Could you check a few things on this model? Use its own coordinates, in mm. Give positions to 0.01 mm unless a question says otherwise; leave off trailing zeros. Loops run counter-clockwise (first coordinate to the right, second up) from the corner with the lowest first, then second, coordinate; pieces in that order, holes last. Notation, with made-up numbers: M 69,13.25 L 96,13.25 A25 ccw 96,50.25 Z; hole C 0.25,43.5 d4. An arc over 180 degrees is marked long. Return JSON: item names as keys, results as strings. Group by question number.
1. If we section it at C-C (z = 2.5): Write out the boundary of the cut face in (x, y).
2. Please list where these lines run through material, in increasing order: line 1 (Y direction, x = 0, z = 1.2); line 2 (Z direction, x = 2.75, y = -1.75); line 3 (Y direction, x = -1.25, z = 0.75).
3. If we section it at D-D (z = 4.5): Write out the boundary of the cut face in (x, y).
4. For pin 1 (1.5 mm diameter, centred on y = -4, z = 2, fed in from -X); pin 2 (2.5 mm diameter, centred on x = -2, y = -1.5, fed in from +Z); pin 3 (1 mm diameter, centred on x = -3, z = 6.5, fed in from -Y), each with a flat end and sliding along its axis, tell me the tip position at first contact or that it passes through.
5. If we section it at A-A (y = 0): Write out the boundary of the cut face in (x, z).
6. If we mould it in two halves opening along X, with no side actions, what happens to faces 1 (the flat face through (0, 0, -1.5)), 2 (the conical face through (3.82, -1.58, 4.91)), 3 (the cylindrical face through (-1.17, -5.26, 3.51))? For each: +X half, -X half, draft (parallel to the pull), parting line (faces both ways), or undercut.
```python
from build123d import *

# Parameters (mm, degrees)
F0_R     = 5.39
F0_R_2   = 3.95
F1_DEPTH = 1.5
F2_DEPTH = 8
F3_SIZE2 = 5
F3_SIZE  = 0.48
F4_SIZE  = 0.4


with BuildPart() as f1:
    # F0 (on Top) → F1 (new body)
    with BuildSketch(Plane.XY):
        Circle(F0_R)
        Circle(F0_R_2, mode=Mode.SUBTRACT)
        Circle(F0_R_2)
    extrude(amount=-F1_DEPTH)

    # F0 (on Top) → F2 (join)
    with BuildSketch(Plane.XY):
        Circle(F0_R)
        Circle(F0_R_2, mode=Mode.SUBTRACT)
    extrude(amount=F2_DEPTH)

    # F3
    f3_edges = [f1.edges().sort_by_distance(p)[0] for p in [
        (-3.95, 0, 8),
    ]]
    chamfer(f3_edges, length=F3_SIZE, length2=F3_SIZE2)

    # F4
    f4_edges = [f1.edges().sort_by_distance(p)[0] for p in [
        (-5.39, 0, -1.5),
    ]]
    chamfer(f4_edges, length=F4_SIZE)


solid = f1.part
```
Answer:
{
 "1": {"outline": "C 0,0 d10.78; hole C 0,0 d7.9"},
 "2": {"line 1": "y = -5.39 to -3.95, 3.95 to 5.39", "line 2": "z = -1.5 to 0", "line 3": "y = -5.24 to -3.75, 3.75 to 5.24"},
 "3": {"outline": "C 0,0 d10.78; hole C 0,0 d8.19"},
 "4": {"pin 1": "stops at x = -4.3", "pin 2": "stops at z = 0", "pin 3": "stops at y = -4.78"},
 "5": {"outline": "M -5.39,-1.1 L -4.99,-1.5 L 4.99,-1.5 L 5.39,-1.1 L 5.39,8 L 4.43,8 L 3.95,3 L 3.95,0 L -3.95,0 L -3.95,3 L -4.43,8 L -5.39,8 Z"},
 "6": {"face 1": "draft", "face 2": "undercut", "face 3": "parting line"}
}
